```python
from build123d import *

# Parameters (mm, degrees)
SALIENTE_EXTRUIR1_DEPTH = 20
CROQUIS2_R              = 40
SALIENTE_EXTRUIR2_DEPTH = 60
CROQUIS3_R              = 30
CORTAR_EXTRUIR1_DEPTH   = 20
CROQUIS4_R              = 20
CORTAR_EXTRUIR2_DEPTH   = 104.923048454
CROQUIS6_W              = 71.704078793
CROQUIS6_H              = 65.206875147
CORTAR_EXTRUIR4_DEPTH   = 117.619037897


with BuildPart() as part:
    # Croquis1 → Saliente-Extruir1 (new body)
    with BuildSketch(Plane(origin=(0, 0, 0), x_dir=(1, 0, 0), z_dir=(0, 1, 0))):
        with BuildLine():
            Line((-30, 60), (30, 60))
            ThreePointArc((30, 60), (51.213203436, 51.213203436), (60, 30))
            Line((60, 30), (60, -30))
            ThreePointArc((60, -30), (51.213203436, -51.213203436), (30, -60))
            Line((30, -60), (-30, -60))
            ThreePointArc((-30, -60), (-51.213203436, -51.213203436), (-60, -30))
            Line((-60, -30), (-60, 30))
            ThreePointArc((-60, 30), (-51.213203436, 51.213203436), (-30, 60))
        make_face()
    extrude(amount=SALIENTE_EXTRUIR1_DEPTH)

    # Croquis2 → Saliente-Extruir2 (add)
    with BuildSketch(Plane(origin=(0, 20, 0), x_dir=(1, 0, 0), z_dir=(0, 1, 0))):
        with Locations(Location((0, 0, 0), (0, 0, 90))):
            Circle(CROQUIS2_R)
    extrude(amount=SALIENTE_EXTRUIR2_DEPTH)

    # Croquis3 → Cortar-Extruir1 (cut)
    with BuildSketch(Plane(origin=(0, 80, 0), x_dir=(1, 0, 0), z_dir=(0, 1, 0))):
        with Locations(Location((0, 0, 0), (0, 0, 270))):
            Circle(CROQUIS3_R)
    extrude(amount=-CORTAR_EXTRUIR1_DEPTH, mode=Mode.SUBTRACT)

    # Croquis4 → Cortar-Extruir2 (cut, through all)
    with BuildSketch(Plane(origin=(0, 60, 0), x_dir=(1, 0, 0), z_dir=(0, 1, 0))):
        with Locations(Location((0, 0, 0), (0, 0, 270))):
            Circle(CROQUIS4_R)
    extrude(amount=-CORTAR_EXTRUIR2_DEPTH, mode=Mode.SUBTRACT)

    # Croquis6 → Cortar-Extruir4 (cut, through all)
    with BuildSketch(Plane(origin=(0, 80, 0), x_dir=(1, 0, 0), z_dir=(0, 1, 0))):
        with Locations((35.852039397, -32.603437574)):
            Rectangle(CROQUIS6_W, CROQUIS6_H)
    extrude(amount=-CORTAR_EXTRUIR4_DEPTH, mode=Mode.SUBTRACT)


solid = part.part
```
Could you check a few things on this model? Use its own coordinates, in mm. A direction names the side the tool comes from. Round coordinates to 2 decimals unless told otherwise and drop trailing zeros. Loops run counter-clockwise (first coordinate to the right, second up) from the corner with the lowest first, then second, coordinate; pieces in that order, holes last. Notation, with made-up numbers: M 34,30 L 92,30 A19 ccw 92,42 Z; hole C 80,13 d5. An arc over 180 degrees is marked long. Write item = value, one per line.
1. I want a section at D-D, the plane x = 22. Write out the boundary of the cut face in (y, z).
Results below:
outline = M 0,-60 L 20,-60 L 20,-33.41 L 80,-33.41 L 80,-20.4 L 60,-20.4 L 60,0 L 0,0 Z
2. I need wall thicknesses on probe 1 along Y at (x, z) = (4.5, -53); probe 2 along Z at (x, y) = (27, 7.5); probe 3 along Z at (x, y) = (-9.5, 69.5). Which ranges of each line are inside material? Lowest first, please.
Results below:
probe_1 = 0 to 20
probe_2 = -60 to 0
probe_3 = -38.86 to -28.46, 28.46 to 38.86
3. Which directions (+Z, -Z, +X, -X, +Y, -Y) give clear straight access to the entire face, cutting with the end or side of a thin tool? Please do faces 1 (the face through (0, 32, 36)), 2 (the face through (-20.502, 70.14, -21.901)), 3 (the face through (50.979, 9.86, -51.445)).
Results below:
face_1 = +Z, +X, +Y, -Y
face_2 = +Y
face_3 = -Z, +X, +Y, -Y
4. I want a section at C-C, the plane y = 8.5. Write out the boundary of the cut face in (x, z).
Results below:
outline = M -60,-30 A30 ccw -30,-60 L 30,-60 A30 ccw 60,-30 L 60,0 L 20,0 A20 cw long 0,20 L 0,60 L -30,60 A30 ccw -60,30 Z
5. I want a section at A-A, the plane x = -4. Write out the boundary of the cut face in (y, z).
Results below:
outline = M 0,-60 L 20,-60 L 20,-39.8 L 80,-39.8 L 80,-29.73 L 60,-29.73 L 60,-19.6 L 0,-19.6 Z; M 0,19.6 L 60,19.6 L 60,29.73 L 80,29.73 L 80,39.8 L 20,39.8 L 20,60 L 0,60 Z
6. Thinking about a two-plate mould opening in Z: for faces 4 (the face through (-15.4, 60, -13.5)), 5 (the face through (-12, 0, -28)), 6 (the face through (-15, 10, 60)), which applies, +Z half, -Z half, draft (parallel to the pull), parting line (faces both ways), or undercut?
Results below:
face_4 = undercut
face_5 = draft
face_6 = +Z half
7. I want a section at B-B, the plane z = -14. Write out the boundary of the cut face in (x, y), and give its area (3 significant figures).
Results below:
outline = M -60,0 L -14.28,0 L -14.28,60 L -26.53,60 L -26.53,80 L -37.47,80 L -37.47,20 L -60,20 Z; M 14.28,0 L 60,0 L 60,20 L 37.47,20 L 37.47,80 L 26.53,80 L 26.53,60 L 14.28,60 Z
area = 4,120 mm²
8. Will these pins go through, and if not, where does the flat tip stop? P1, Ø5, axis at x = 32, z = -36.5, coming from the +Y side; P2, Ø10, axis at x = 36, y = 32, coming from the -Z side; P3, Ø4, axis at x = -37, y = 23, coming from the +Z side; P4, Ø24, axis at x = 0, z = 0, coming from the -Y side.
Results below:
P1 = 20
P2 = -25.28
P3 = 19.36
P4 = through
